For this review, take the finished solid that the model builds, in its own axes (mm). Face numbers are marked on the shaded views. A direction names the side the tool comes from. Round coordinates to 2 decimals unless told otherwise and drop trailing zeros. Loops run counter-clockwise (first coordinate to the right, second up) from the corner with the lowest first, then second, coordinate; pieces in that order, holes last.
1. Clearance check with flat-ended pins moving along their axes: pin 1 Ø8 at (y, z) = (25.5, 2.5) entering from -X; pin 2 Ø8 at (x, z) = (-36.5, 4.5) entering from +Y; pin 3 Ø6 at (x, z) = (24.5, 3.5) entering from -Y; pin 4 Ø1 at (y, z) = (-25.5, 9) entering from +X. State where each tip first meets the part, or that it passes through.
2. To check wall thickness, follow line 1 along Z through (x, y) = (23.5, 4); line 2 along X through (y, z) = (-27, 1.5). State the ranges of each line that lie inside material, in increasing order.
3. Consider section A-A on z = 6. State the section outline as (x, y) points, then the cut area to 3 significant figures.
4. Consider section B-B on y = 38.5. State the section outline as (x, z) points, then the cut area to 3 significant figures.
5. Tool access review of the marked faces 1, 2 and 3: name each direction out of +Z, -Z, +X, -X, +Y, -Y from which nothing blocks a thin tool from reaching the whole face with its end or side.
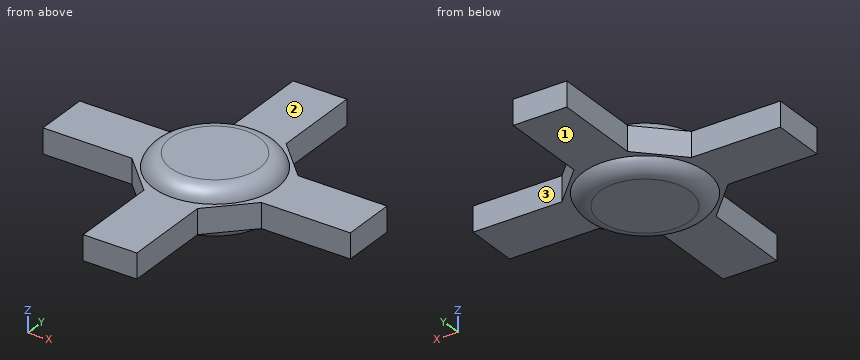
from build123d import *

# Parameters (mm, degrees)
F1_DEPTH = 7.112
F2_DEPTH = 25.4
F3_DEPTH = 25.4
F4_DEPTH = 25.4
F5_DEPTH = 25.4
F6_R     = 17.6209063201
F7_DEPTH = 10.922
F8_DEPTH = 3.556


# Not quite as in the source:
# - a fillet or chamfer that OpenCascade refuses, or shapes differently, is made with other operations: its cross-section is extruded or revolved along the edge and cut away or added


with BuildPart() as f1:
    # F0 (on Top) → F1 (new body)
    with BuildSketch(Plane.XY):
        Polygon((7.6623515216, 18.4985529631), (-7.6623515216, 18.4985529631), (-18.4985529631, 7.6623515216), (-18.4985529631, -7.6623515216), (-7.6623515216, -18.4985529631), (7.6623515216, -18.4985529631), (18.4985529631, -7.6623515216), (18.4985529631, 7.6623515216), align=None)
    extrude(amount=F1_DEPTH)

    # F2 (add): a face of the model
    f2_faces = [f1.faces().sort_by_distance(p)[0] for p in [
        (0, -18.4985529631, 3.556),
    ]]
    extrude(f2_faces, amount=F2_DEPTH)

    # F3 (add): a face of the model
    f3_faces = [f1.faces().sort_by_distance(p)[0] for p in [
        (-18.4985529631, 0, 3.556),
    ]]
    extrude(f3_faces, amount=F3_DEPTH)

    # F4 (add): a face of the model
    f4_faces = [f1.faces().sort_by_distance(p)[0] for p in [
        (0, 18.4985529631, 3.556),
    ]]
    extrude(f4_faces, amount=F4_DEPTH)

    # F5 (add): a face of the model
    f5_faces = [f1.faces().sort_by_distance(p)[0] for p in [
        (18.4985529631, 0, 3.556),
    ]]
    extrude(f5_faces, amount=F5_DEPTH)

    # F6 (on Top) → F7 (join)
    with BuildSketch(Plane.XY):
        Circle(F6_R)
    extrude(amount=F7_DEPTH)

    # F6 (on Top) → F8 (join)
    with BuildSketch(Plane.XY):
        Circle(F6_R)
    extrude(amount=-F8_DEPTH)

    # F9: fillet of radius 5.08 on 1 edges, made by hand

    # F9_s1 → F9_t2 (revolve, cut)
    with BuildSketch(Plane.XZ):
        with BuildLine():
            ThreePointArc((17.6209063201, 7.112), (15.8130694437, 9.8580926284), (12.7022174704, 10.922))
            Line((12.7022174704, 10.922), (17.6209063201, 10.922))
            Line((17.6209063201, 10.922), (17.6209063201, 7.112))
        make_face()
    revolve(axis=Axis((0, 0, 10.922), (0, 0, 1)), mode=Mode.SUBTRACT)

    # F10: fillet of radius 5.08 on 1 edges, made by hand

    # F10_s1 → F10_t2 (revolve, cut)
    with BuildSketch(Plane.XZ):
        with BuildLine():
            ThreePointArc((17.6209063201, 0), (15.7802637067, -2.5716269361), (12.7748951769, -3.556))
            Line((12.7748951769, -3.556), (17.6209063201, -3.556))
            Line((17.6209063201, -3.556), (17.6209063201, 0))
        make_face()
    revolve(axis=Axis((0, 0, -3.556), (0, 0, 1)), mode=Mode.SUBTRACT)


solid = f1.part
Resolved:
1. pin 1: stops at x = -7.66
1. pin 2: stops at y = 7.66
1. pin 3: stops at y = -7.66
1. pin 4: passes through
2. line 1: z = 0 to 7.11
2. line 2: x = -7.66 to 7.66
3. outline: (-43.9, -7.66) - (-18.5, -7.66) - (-7.66, -18.5) - (-7.66, -43.9) - (7.66, -43.9) - (7.66, -18.5) - (18.5, -7.66) - (43.9, -7.66) - (43.9, 7.66) - (18.5, 7.66) - (7.66, 18.5) - (7.66, 43.9) - (-7.66, 43.9) - (-7.66, 18.5) - (-18.5, 7.66) - (-43.9, 7.66) - close
3. area: 2,690 mm2
4. outline: (-7.66, 0) - (7.66, 0) - (7.66, 7.11) - (-7.66, 7.11) - close
4. area: 109 mm2
5. face 1: -Z
5. face 2: +Z
5. face 3: +Z, -Z, +X, +Y
